```python
from build123d import *

# Parameters (mm, degrees)
F2_R     = 9.525
F3_DEPTH = 7.7216


with BuildPart() as f1:
    # F0 (on Right) → F1 (revolve)
    with BuildSketch(Plane.YZ):
        Polygon((0, 7.14375), (0, 0), (43.18, 0), (43.18, 0.635), (37.5158, 0.635), (37.5158, 2.5019), (9.5504, 2.5019), (9.5504, 7.14375), align=None)
    revolve(axis=Axis((0, -1.133929, 0), (0, -1, 0)))

    # F2 (on face) → F3 (cut)
    with BuildSketch(Plane.XZ):
        Circle(F2_R)
    extrude(amount=-F3_DEPTH, mode=Mode.SUBTRACT)


solid = f1.part
```
Design review of the part built by this model. Coordinates are the model's own, in mm. A direction names the side the tool comes from. Give positions to 0.01 mm unless a question says otherwise; leave off trailing zeros. Loops run counter-clockwise (first coordinate to the right, second up) from the corner with the lowest first, then second, coordinate; pieces in that order, holes last. Notation, with made-up numbers: M 87.25,-30 L 141.25,-30 A20 cw 141.25,-7 Z; hole C -33,62.5 d7. An arc over 180 degrees is marked long. Return JSON: item names as keys, results as strings. Group by question number.
Item 1: We need section D-D (x = 1.5). Give the boundary of the cut face in (y, z), and give its area (3 significant figures).
Item 2: Insertion check: pin 1 Ø1.5 at (x, z) = (-3, -2) entering from +Y; pin 2 Ø8 at (x, y) = (-3, 37.5) entering from -Z; pin 3 Ø8 at (y, z) = (15, 5) entering from +X; pin 4 Ø7 at (x, z) = (2, -3.5) entering from +Y. Each pin has a flat end and moves straight along its axis. Give the tip position at first contact, or say it passes through.
Item 3: We need section A-A (x = 0). Give the boundary of the cut face in (y, z) (3 decimals), and give its area (3 significant figures).
Item 4: For probe 1 along Y at (x, z) = (0.5, -4); probe 2 along Y at (x, z) = (0.5, -2); probe 3 along Z at (x, y) = (-0.5, 38.5), list the stretches that pass through material, from the lowest coordinate up.
Item 5: We need section C-C (y = 39.5). Give the boundary of the cut face in (x, z) (3 decimals).
Item 6: We need section B-B (z = 0). Give the boundary of the cut face in (x, y) (3 decimals), and give its area (3 significant figures).
Item 7: Tool access review of faces 1 (the flat face through (1, 37.516, -1)), 2 (the flat face through (0, 43.18, 0)): name each direction out of +Z, -Z, +X, -X, +Y, -Y from which nothing blocks a thin tool from reaching the whole face with its end or side.
Output:
{
 "1": {"outline": "M 7.72,-6.98 L 9.55,-6.98 L 9.55,-2 L 37.52,-2 L 37.52,2 L 9.55,2 L 9.55,6.98 L 7.72,6.98 Z", "area": "138 mm^2"},
 "2": {"pin 1": "stops at y = 9.55", "pin 2": "stops at z = -2.5", "pin 3": "stops at x = 2.29", "pin 4": "stops at y = 43.18"},
 "3": {"outline": "M 7.722,-7.144 L 9.55,-7.144 L 9.55,-2.502 L 37.516,-2.502 L 37.516,-0.635 L 43.18,-0.635 L 43.18,0.635 L 37.516,0.635 L 37.516,2.502 L 9.55,2.502 L 9.55,7.144 L 7.722,7.144 Z", "area": "173 mm^2"},
 "4": {"probe 1": "y = 7.72 to 9.55", "probe 2": "y = 7.72 to 37.52", "probe 3": "z = -0.39 to 0.39"},
 "5": {"outline": "C 0,0 d1.27"},
 "6": {"outline": "M -7.144,7.722 L 7.144,7.722 L 7.144,9.55 L 2.502,9.55 L 2.502,37.516 L 0.635,37.516 L 0.635,43.18 L -0.635,43.18 L -0.635,37.516 L -2.502,37.516 L -2.502,9.55 L -7.144,9.55 Z", "area": "173 mm^2"},
 "7": {"face 1": "+Y", "face 2": "+Z, -Z, +X, -X, +Y"}
}
